```python
from build123d import *

# Parameters (mm, degrees)
SKETCH1_W               = 635
SKETCH1_H               = 101.6
BOSS_EXTRUDE1_DEPTH     = 32.512
CUT_EXTRUDE2_START      = -33.512
SKETCH1_3_R             = 14.2875
CUT_EXTRUDE2_DEPTH      = 34.512
LPATTERN1_COUNT         = 17
LPATTERN1_PITCH         = 34.925
SKETCH3_R               = 14.2875
CUT_EXTRUDE3_DEPTH      = 1
CUT_EXTRUDE3_DEPTH_BACK = 33.512


with BuildPart() as part:
    # Sketch1 → Boss-Extrude1 (new body)
    with BuildSketch(Plane.XY):
        with Locations((-279.4, 0.08382)):
            Rectangle(SKETCH1_W, SKETCH1_H)
    extrude(amount=-BOSS_EXTRUDE1_DEPTH)

    # Sketch1<3> → Cut-Extrude2 (cut)
    with BuildSketch(Plane.XY.offset(CUT_EXTRUDE2_START)):
        Circle(SKETCH1_3_R)
        with Locations((17.4625, 30.24632)):
            Circle(SKETCH1_3_R)
        with Locations((17.4625, -30.24632)):
            Circle(SKETCH1_3_R)
    cut_extrude2 = extrude(amount=CUT_EXTRUDE2_DEPTH, mode=Mode.SUBTRACT)

    # LPattern1: Cut-Extrude2 ×17
    with Locations(*[(-i * LPATTERN1_PITCH, 0, 0) for i in range(1, LPATTERN1_COUNT)]):
        add(cut_extrude2, mode=Mode.SUBTRACT)

    # Sketch3 → Cut-Extrude3 (cut, two sides)
    with BuildSketch(Plane.XY) as cut_extrude3_sk:
        with Locations((-576.2625, 30.24632)):
            Circle(SKETCH3_R)
        with Locations((-576.2625, -30.24632)):
            Circle(SKETCH3_R)
    extrude(amount=CUT_EXTRUDE3_DEPTH, mode=Mode.SUBTRACT)
    extrude(cut_extrude3_sk.sketch, amount=-CUT_EXTRUDE3_DEPTH_BACK, mode=Mode.SUBTRACT)


solid = part.part
```
Geometry: final body of the model. Coordinates: model frame, mm. Round coordinates to 2 decimals unless told otherwise and drop trailing zeros. Order: outer loops, then holes, each group sorted by start corner. A loop starts at its lowest first (then second) coordinate and runs counter-clockwise, first axis right, second up. Notation, with made-up numbers: (39.5, -25) -> (83.5, -25) arc R33 ccw to (83.5, 4) -> close; hole circle Ø11 at (-11.75, 10). An arc over 180 degrees is marked (long way). Use one line per item in the form item = value. Start each with the question number.
1. Line query: probe 1 along Y at (x, z) = (0, -16); probe 2 along Y at (x, z) = (-23.5, -14); probe 3 along Y at (x, z) = (-400, -3). Output: solid intervals per line, ascending.
2. Cut plane B-B (y = 0). Count the separate pieces of the cut face and the enclosed holes in it, then the cut area to 3 significant figures.
3. Draft query along Y for faces 1 (the face through (-328.6, 0.6, -16.5)), 2 (the face through (-284, 50.884, -16)), 3 (the face through (-284, -50.716, -16)). Return one class per face: pulls with the +Y half, pulls with the -Y half, needs draft (parallel to the pull), parting line crosses it, or undercut.
4. Pin query (flat end, axial travel): pin 1 Ø6 at (x, y) = (-480, 21.5) entering from -Z. Return the tip coordinate at first contact, or that it passes through.
5. Cut plane A-A (x = -393). Return the cut outline in (y, z).
Solution:
q1.probe_1 = -50.72 to -14.29, 14.29 to 50.88
q1.probe_2 = -50.72 to -43.2, -17.3 to -8.58, 8.58 to 17.3, 43.2 to 50.88
q1.probe_3 = -50.72 to -44.44, -16.05 to 16.05, 44.44 to 50.88
q2.separate_pieces = 18
q2.enclosed_holes = 0
q2.area = 4,850 mm^2
q3.face_1 = undercut
q3.face_2 = pulls with the +Y half
q3.face_3 = pulls with the -Y half
q4.pin_1 = -32.51
q5.outline = (-50.72, -32.51) -> (-41.63, -32.51) -> (-41.63, 0) -> (-50.72, 0) -> close; (-18.87, -32.51) -> (-11.24, -32.51) -> (-11.24, 0) -> (-18.87, 0) -> close; (11.24, -32.51) -> (18.87, -32.51) -> (18.87, 0) -> (11.24, 0) -> close; (41.63, -32.51) -> (50.88, -32.51) -> (50.88, 0) -> (41.63, 0) -> close
